Here's how the part is built. I have some questions about the finished solid (model axes, mm). A direction names the side the tool comes from. Give positions to 0.01 mm unless a question says otherwise; leave off trailing zeros. Loops run counter-clockwise (first coordinate to the right, second up) from the corner with the lowest first, then second, coordinate; pieces in that order, holes last.
Q1. If we section it at C-C (x = 9.5): Give the number of separate pieces and of enclosed holes in the cut face, plus the area to 3 significant figures.
Q2. We'd pull the mould along Z, two halves only. Please class faces 1 (the face through (5.916, 160.393, 347.872)), 2 (the face through (6, 33, 5)), 3 (the face through (6, 45, -32)): +Z half, -Z half, draft (parallel to the pull), parting line (faces both ways), or undercut.
Q3. If we section it at D-D (z = 380.5): Please give me the cut outline in (x, y), plus the area to 3 significant figures.
Q4. Will these pins go through, and if not, where does the flat tip stop? P1, Ø3.5, axis at x = 5, z = 7, coming from the +Y side; P2, Ø3.5, axis at x = 3, y = 38, coming from the +Z side; P3, Ø3.5, axis at x = 8, y = 36, coming from the -Z side.
Q5. If we section it at A-A (z = -108.5): Please give me the cut outline in (x, y).
Q6. If we section it at B-B (z = 287.5): Please give me the cut outline in (x, y).
Q7. I need wall thicknesses on line 1 (Y direction, x = 8.75, z = -90); line 2 (Z direction, x = 3, y = 0); line 3 (Y direction, x = 7, z = 28.5). Which ranges of each line are inside material? Lowest first, please.
Q8. For faces 4 (the face through (6, 45, -104)), 5 (the face through (6, -75, -104)), 6 (the face through (5.916, -70.495, -58.221)), 7 (the face through (6, 39, -121.478)), 8 (the face through (6.084, 127.358, 224.585)), which set-ups out of +Z, -Z, +X, -X, +Y, -Y let a thin tool reach every point of the face, with its end or its side?
Autodesk Inventor part; units mm, degrees
ref_plane "YZ Plane" through (0, 0, 0) normal (1, 0, 0) x (0, 1, 0)
ref_plane "XZ Plane" through (0, 0, 0) normal (0, 1, 0) x (-1, 0, 0)
ref_plane "XY Plane" through (0, 0, 0) normal (0, 0, 1) x (1, 0, 0)
sketch "Sketch1" plane through (0, 0, 0) normal (1, 0, 0) x (0, 1, 0)
  circle A0 centre (0, 316.1768) radius 4
  line L0 (0, -83.8232) -> (0, -123.8232)
  line L1 (-4, -83.8232) -> (-4, -123.8232)
  line L2 (4, -123.8232) -> (4, -83.8232)
  arc A1 (4, -83.8232) -> (-4, -83.8232) centre (0, -83.8232) ccw
  arc A2 (-4, -123.8232) -> (4, -123.8232) centre (0, -123.8232) ccw
  arc A3 (29.4615, 385.1479) -> (-59.8687, 271.0022) centre (0, 316.1768) ccw construction
  line L3 (-75, -123.8232) -> (-75, -83.8232) construction
  line L4 (45, -142.4909) -> (45, -229.6533) construction
  arc A4 (-75, -123.8232) -> (-37.5, -188.7751) centre (0, -123.8232) ccw construction
  circle A5 centre (0, 316.1768) radius 115 construction
  line L5 (-115, -63.8232) -> (-115, -123.8232) construction
  arc A6 (-115, -123.8232) -> (115, -123.8232) centre (0, -123.8232) ccw construction
  line L6 (115, -123.8232) -> (115, -63.8232) construction
  arc A7 (115, -63.8232) -> (-115, -63.8232) centre (0, -83.8232) ccw construction
  line L7 (111.5189, 432.5238) -> (211.5189, 259.3187)
  line L8 (211.5189, 259.3187) -> (45, 163.179)
  circle A8 centre (0, 316.1768) radius 45 construction
  arc A9 (29.4615, 385.1479) -> (-59.8687, 271.0022) centre (0, 316.1768) ccw
  line L9 (-75, -123.8232) -> (-75, -83.8232)
  arc A10 (-57.0417, -35.1278) -> (-75, -83.8232) centre (0, -83.8232) ccw
  arc A11 (-75, -123.8232) -> (-37.5, -188.7751) centre (0, -123.8232) ccw
  line L10 (-46.3992, 230.789) -> (-46.3992, -6.2697)
  arc A12 (-46.3992, 230.789) -> (-59.8687, 271.0022) centre (-113.1622, 230.789) ccw
  arc A13 (-57.0417, -35.1278) -> (-46.3992, -6.2697) centre (-90.846, -6.2697) ccw
  line L11 (45, -229.4783) -> (45, 163.179)
  line L12 (43.5102, 150.8148) -> (13.9439, 202.0253) construction
  line L13 (-38.9711, 293.6768) -> (-61.4711, 332.6479) construction
  line L14 (-61.4711, 332.6479) -> (-22.5, 355.1479) construction
  line L15 (29.4615, 385.1479) -> (111.5189, 432.5238)
  line L16 (45, -229.4783) -> (33, -229.4783)
  line L17 (33, -229.4783) -> (-37.5, -188.7751)
  line L18 (45, 316.1768) -> (45, 281.1768) construction
  line L19 (-75, -123.8232) -> (-75, -83.8232) construction
  arc A14 (75, -83.8232) -> (-75, -83.8232) centre (0, -83.8232) ccw construction
  line L20 (75, -83.8232) -> (75, -123.8232) construction
  arc A15 (-75, -123.8232) -> (75, -123.8232) centre (0, -123.8232) ccw construction
  point P0 (0, 0)
  point P1 (0, -103.8232)
  dimension "d7" = 230
  dimension "d0" = 8
  dimension "d1" = 8
  dimension "d2" = 400
  dimension "d3" = 40
  dimension "d5" = 150
  dimension "d8" = 115
  dimension "d9" = 200
  dimension "d10" = 200
  dimension "d12" = 90
  dimension "d13" = 12
  dimension "d15" = 120
  dimension "d16" = 120
  dimension "d17" = 75
extrude "Extrusion1" add sketch "Sketch1" along normal blind 12
fillet "Fillet1" radius 100 1 edges at (6, 29.4615, 385.1479)
sketch "Sketch2" plane through (12, 0, 0) normal (1, 0, 0) x (0, 0, -1)
  line L0 (229.4783, 45) -> (-163.179, 45) construction
  line L1 (229.4783, 45) -> (193.4783, 45)
  line L2 (193.4783, 45) -> (193.4783, 33)
  line L3 (193.4783, 33) -> (229.4783, 33)
  line L4 (229.4783, 33) -> (229.4783, 45)
  line L5 (-163.179, 45) -> (-259.3187, 211.5189) construction
  line L6 (-432.5238, 111.5189) -> (-404.1377, 62.3528) construction
  line L7 (-259.3187, 211.5189) -> (-432.5238, 111.5189) construction
  line L8 (-432.5238, 111.5189) -> (-332.5238, -61.6862) construction
  line L9 (-332.5238, -61.6862) -> (-159.3187, 38.3138) construction
  line L10 (-159.3187, 38.3138) -> (-259.3187, 211.5189) construction
  line L11 (-259.3187, 211.5189) -> (-241.3187, 180.342)
  line L12 (-241.3187, 180.342) -> (-251.711, 174.342)
  line L13 (-251.711, 174.342) -> (-269.711, 205.5189)
  line L14 (-269.711, 205.5189) -> (-259.3187, 211.5189)
  line L15 (-432.5238, 111.5189) -> (-159.3187, 38.3138) construction
  line L16 (193.4783, 45) -> (157.4783, 45)
  line L17 (157.4783, 33) -> (193.4783, 33)
  line L18 (193.4783, 33) -> (193.4783, 45)
  line L19 (157.4783, 45) -> (157.4783, 33)
  line L20 (157.4783, 45) -> (121.4783, 45)
  line L21 (121.4783, 33) -> (157.4783, 33)
  line L22 (157.4783, 33) -> (157.4783, 45)
  line L23 (121.4783, 45) -> (121.4783, 33)
  line L24 (121.4783, 45) -> (85.4783, 45)
  line L25 (85.4783, 33) -> (121.4783, 33)
  line L26 (121.4783, 33) -> (121.4783, 45)
  line L27 (85.4783, 45) -> (85.4783, 33)
  line L28 (85.4783, 45) -> (49.4783, 45)
  line L29 (49.4783, 33) -> (85.4783, 33)
  line L30 (85.4783, 33) -> (85.4783, 45)
  line L31 (49.4783, 45) -> (49.4783, 33)
  line L32 (49.4783, 45) -> (13.4783, 45)
  line L33 (13.4783, 33) -> (49.4783, 33)
  line L34 (49.4783, 33) -> (49.4783, 45)
  line L35 (13.4783, 45) -> (13.4783, 33)
  line L36 (13.4783, 45) -> (-22.5217, 45)
  line L37 (-22.5217, 33) -> (13.4783, 33)
  line L38 (13.4783, 33) -> (13.4783, 45)
  line L39 (-22.5217, 45) -> (-22.5217, 33)
  line L40 (-22.5217, 45) -> (-58.5217, 45)
  line L41 (-58.5217, 33) -> (-22.5217, 33)
  line L42 (-22.5217, 33) -> (-22.5217, 45)
  line L43 (-58.5217, 45) -> (-58.5217, 33)
  line L44 (-58.5217, 45) -> (-94.5217, 45)
  line L45 (-94.5217, 33) -> (-58.5217, 33)
  line L46 (-58.5217, 33) -> (-58.5217, 45)
  line L47 (-94.5217, 45) -> (-94.5217, 33)
  line L48 (-94.5217, 45) -> (-130.5217, 45)
  line L49 (-130.5217, 33) -> (-94.5217, 33)
  line L50 (-94.5217, 33) -> (-94.5217, 45)
  line L51 (-130.5217, 45) -> (-130.5217, 33)
  line L52 (-130.5217, 45) -> (-166.5217, 45)
  line L53 (-166.5217, 33) -> (-130.5217, 33)
  line L54 (-130.5217, 33) -> (-130.5217, 45)
  line L55 (-166.5217, 45) -> (-166.5217, 33)
  line L56 (-166.5217, 45) -> (-202.5217, 45)
  line L57 (-202.5217, 33) -> (-166.5217, 33)
  line L58 (-166.5217, 33) -> (-166.5217, 45)
  line L59 (-202.5217, 45) -> (-202.5217, 33)
  line L60 (-251.711, 174.342) -> (-241.3187, 180.342)
  line L61 (-233.711, 143.1651) -> (-251.711, 174.342)
  line L62 (-241.3187, 180.342) -> (-223.3187, 149.1651)
  line L63 (-223.3187, 149.1651) -> (-233.711, 143.1651)
  line L64 (-233.711, 143.1651) -> (-223.3187, 149.1651)
  line L65 (-215.711, 111.9882) -> (-233.711, 143.1651)
  line L66 (-223.3187, 149.1651) -> (-205.3187, 117.9882)
  line L67 (-205.3187, 117.9882) -> (-215.711, 111.9882)
  line L68 (-215.711, 111.9882) -> (-205.3187, 117.9882)
  line L69 (-197.711, 80.8112) -> (-215.711, 111.9882)
  line L70 (-205.3187, 117.9882) -> (-187.3187, 86.8112)
  line L71 (-187.3187, 86.8112) -> (-197.711, 80.8112)
  line L72 (-197.711, 80.8112) -> (-187.3187, 86.8112)
  line L73 (-179.711, 49.6343) -> (-197.711, 80.8112)
  line L74 (-187.3187, 86.8112) -> (-169.3187, 55.6343)
  line L75 (-169.3187, 55.6343) -> (-179.711, 49.6343)
  line L76 (-259.3187, 211.5189) -> (-432.5238, 111.5189)
  line L77 (-269.711, 205.5189) -> (-300.8879, 187.5189)
  line L78 (-300.8879, 187.5189) -> (-294.8879, 177.1266)
  line L79 (-294.8879, 177.1266) -> (-263.711, 195.1266)
  line L80 (-263.711, 195.1266) -> (-269.711, 205.5189)
  line L81 (-294.8879, 177.1266) -> (-300.8879, 187.5189)
  line L82 (-326.0648, 159.1266) -> (-294.8879, 177.1266)
  line L83 (-300.8879, 187.5189) -> (-332.0648, 169.5189)
  line L84 (-332.0648, 169.5189) -> (-326.0648, 159.1266)
  line L85 (-290.4956, 193.5189) -> (-463.7007, 93.5189) construction
  line L86 (-326.0648, 159.1266) -> (-332.0648, 169.5189)
  line L87 (-357.2417, 141.1266) -> (-326.0648, 159.1266)
  line L88 (-332.0648, 169.5189) -> (-363.2417, 151.5189)
  line L89 (-363.2417, 151.5189) -> (-357.2417, 141.1266)
  line L90 (-321.6725, 175.5189) -> (-494.8776, 75.5189) construction
  line L91 (-357.2417, 141.1266) -> (-363.2417, 151.5189)
  line L92 (-388.4187, 123.1266) -> (-357.2417, 141.1266)
  line L93 (-363.2417, 151.5189) -> (-394.4187, 133.5189)
  line L94 (-394.4187, 133.5189) -> (-388.4187, 123.1266)
  line L95 (-352.8494, 157.5189) -> (-526.0545, 57.5189) construction
  line L96 (-388.4187, 123.1266) -> (-394.4187, 133.5189)
  line L97 (-419.5956, 105.1266) -> (-388.4187, 123.1266)
  line L98 (-394.4187, 133.5189) -> (-425.5956, 115.5189)
  line L99 (-425.5956, 115.5189) -> (-419.5956, 105.1266)
  line L100 (-384.0264, 139.5189) -> (-557.2314, 39.5189) construction
  line L101 (-232.0648, -3.6862) -> (-263.2417, -21.6862)
  line L102 (-263.2417, -21.6862) -> (-269.2417, -11.2939)
  line L103 (-269.2417, -11.2939) -> (-238.0648, 6.7061)
  line L104 (-238.0648, 6.7061) -> (-232.0648, -3.6862)
  circle A0 centre (-276.1768, 40) radius 30
  circle A1 centre (-316.1768, 0) radius 4
  point P0 (-295.9212, 74.9164)
  dimension "d21" = 12
  dimension "d22" = 36
  dimension "d26" = 200
  dimension "d27" = 12
  dimension "d28" = 36
  dimension "d31" = 36
  dimension "d38" = 36
  dimension "d45" = 12
  dimension "d46" = 36
  dimension "d49" = 36
  dimension "d54" = 60
  dimension "d55" = 40
  dimension "d56" = 40
  dimension "d57" = 12
extrude "Extrusion2" cut sketch "Sketch2" against normal blind 12 contours L4 L3 L2 L1 | L19 L21 L23 L20 | L27 L29 L31 L28 | L35 L37 L39 L36 | L43 L45 L47 L44 | L11 L12 L13 L14 | L66 L67 L65 L63 | L78 L82 L84 L76 | L74 L75 L73 L71 | L89 L92 L94 L76 | L101 L102 L103 L104 | A0
sketch "Sketch3" plane through (12, 0, 0) normal (1, 0, 0) x (0, 0, -1)
  line L0 (-326.0648, 159.1266) -> (-332.0648, 169.5189)
  line L1 (-332.0648, 169.5189) -> (-363.2417, 151.5189)
  line L2 (-363.2417, 151.5189) -> (-357.2417, 141.1266)
  line L3 (-357.2417, 141.1266) -> (-388.4187, 123.1266)
  line L4 (-388.4187, 123.1266) -> (-394.4187, 133.5189)
  line L5 (-394.4187, 133.5189) -> (-432.5238, 111.5189)
  line L6 (-432.5238, 111.5189) -> (-404.1377, 62.3528)
  arc A0 (-390.9897, 5.2941) -> (-404.1377, 62.3528) centre (-490.7403, 12.3528) ccw
  arc A1 (-390.9897, 5.2941) -> (-271.0022, -59.8687) centre (-316.1768, 0) ccw
  arc A2 (-230.789, -46.3992) -> (-271.0022, -59.8687) centre (-230.789, -113.1622) ccw
  line L7 (-230.789, -46.3992) -> (6.2697, -46.3992)
  arc A3 (35.1278, -57.0417) -> (6.2697, -46.3992) centre (6.2697, -90.846) ccw
  arc A4 (35.1278, -57.0417) -> (83.8232, -75) centre (83.8232, 0) ccw
  line L8 (83.8232, -75) -> (123.8232, -75)
  arc A5 (123.8232, -75) -> (188.7751, -37.5) centre (123.8232, 0) ccw
  line L9 (188.7751, -37.5) -> (229.4783, 33)
  line L10 (229.4783, 33) -> (193.4783, 33)
  line L11 (193.4783, 33) -> (193.4783, 45)
  line L12 (193.4783, 45) -> (157.4783, 45)
  line L13 (157.4783, 45) -> (157.4783, 33)
  line L14 (157.4783, 33) -> (121.4783, 33)
  line L15 (121.4783, 33) -> (121.4783, 45)
  line L16 (121.4783, 45) -> (85.4783, 45)
  line L17 (85.4783, 45) -> (85.4783, 33)
  line L18 (85.4783, 33) -> (49.4783, 33)
  line L19 (49.4783, 33) -> (49.4783, 45)
  line L20 (49.4783, 45) -> (13.4783, 45)
  line L21 (13.4783, 45) -> (13.4783, 33)
  line L22 (13.4783, 33) -> (-22.5217, 33)
  line L23 (-22.5217, 33) -> (-22.5217, 45)
  line L24 (-22.5217, 45) -> (-58.5217, 45)
  line L25 (-58.5217, 45) -> (-58.5217, 33)
  line L26 (-58.5217, 33) -> (-94.5217, 33)
  line L27 (-94.5217, 33) -> (-94.5217, 45)
  line L28 (-94.5217, 45) -> (-163.179, 45)
  line L29 (-163.179, 45) -> (-169.3187, 55.6343)
  line L30 (-169.3187, 55.6343) -> (-179.711, 49.6343)
  line L31 (-179.711, 49.6343) -> (-197.711, 80.8112)
  line L32 (-197.711, 80.8112) -> (-187.3187, 86.8112)
  line L33 (-187.3187, 86.8112) -> (-205.3187, 117.9882)
  line L34 (-205.3187, 117.9882) -> (-215.711, 111.9882)
  line L35 (-215.711, 111.9882) -> (-233.711, 143.1651)
  line L36 (-233.711, 143.1651) -> (-223.3187, 149.1651)
  line L37 (-223.3187, 149.1651) -> (-241.3187, 180.342)
  line L38 (-241.3187, 180.342) -> (-251.711, 174.342)
  line L39 (-251.711, 174.342) -> (-269.711, 205.5189)
  line L40 (-269.711, 205.5189) -> (-300.8879, 187.5189)
  line L41 (-300.8879, 187.5189) -> (-294.8879, 177.1266)
  line L42 (-294.8879, 177.1266) -> (-326.0648, 159.1266)
  line L43 (-238.0648, 6.7061) -> (-232.0648, -3.6862)
  line L44 (-232.0648, -3.6862) -> (-263.2417, -21.6862)
  line L45 (-263.2417, -21.6862) -> (-269.2417, -11.2939)
  line L46 (-269.2417, -11.2939) -> (-238.0648, 6.7061)
  circle A6 centre (-276.1768, 40) radius 30
  line L47 (83.8232, 4) -> (123.8232, 4)
  arc A7 (123.8232, -4) -> (123.8232, 4) centre (123.8232, 0) ccw
  line L48 (123.8232, -4) -> (83.8232, -4)
  arc A8 (83.8232, 4) -> (83.8232, -4) centre (83.8232, 0) ccw
  circle A9 centre (-316.1768, 0) radius 4
  point P0 (0, 0)
equation "\"d8\" = 0.5 * d7"
equation "\"wood_thickness\" = 12"
properties part number "wooden_side"
Check sheet entries:
1. separate pieces: 1
1. enclosed holes: 4
1. area: 79,600 mm2
2. face 1: +Z half
2. face 2: undercut
2. face 3: draft
3. outline: (0, -38.57) - (12, -38.57) - (12, 127.7) - (0, 127.7) - close
3. area: 2,000 mm2
4. P1: stops at y = 33
4. P2: stops at z = 394.57
4. P3: stops at z = -193.48
5. outline: (0, -75) - (12, -75) - (12, -4) - (0, -4) - close; (0, 4) - (12, 4) - (12, 45) - (0, 45) - close
6. outline: (0, -69.3) - (12, -69.3) - (12, 12.22) - (0, 12.22) - close; (0, 67.78) - (12, 67.78) - (12, 195.25) - (0, 195.25) - close
7. line 1: y = -75 to -4, 4 to 45
7. line 2: z = -210.43 to -127.82, -79.82 to 234.19, 249.68 to 312.18, 320.18 to 391.18
7. line 3: y = -46.4 to 45
8. face 4: -Z, +X, -X, +Y
8. face 5: +Z, -Z, +X, -X, -Y
8. face 6: +X, -X, -Y
8. face 7: +X, -X, +Y
8. face 8: +X, -X
